```python
from build123d import *

# Parameters (mm, degrees)
BASPROSKE_W        = 10
BASPROSKE_H        = 22.5
TOOTHCUT_DEPTH     = 34.35416016
TEETHCUTS_COUNT    = 28
TEETHCUTS_ANGLE    = 347.142857143
BORSKE_R           = 7.5
BORE_DEPTH         = 50.0000508
CROQUIS1_OUTSIDE_W = 59.636
CROQUIS1_OUTSIDE_H = 59.636
EXTRUIR1_DEPTH     = 10
CROQUIS2_R         = 7.5
CROQUIS2_R_2       = 3.1
EXTRUIR2_DEPTH     = 10
REDONDEO1_R        = 3


with BuildPart() as part:
    # BasProSke → Base-Revolve (revolve)
    with BuildSketch(Plane(origin=(0, 0, 0), x_dir=(1, 0, 0), z_dir=(0, 1, 0)), mode=Mode.PRIVATE) as base_revolve_sk:
        with Locations((5, 11.25)):
            Rectangle(BASPROSKE_W, BASPROSKE_H)
    revolve(base_revolve_sk.sketch.rotate(Axis((-10, 0, 0), (1, 0, 0)), 180), axis=Axis((-10, 0, 0), (1, 0, 0)))

    # TooCutSke → ToothCut (cut, through all)
    with BuildSketch(Plane(origin=(0, 0, 0), x_dir=(0, 0, -1), z_dir=(1, 0, 0))):
        with BuildLine():
            ThreePointArc((0.70071741, 19.111158288), (0, 19.124), (-0.70071741, 19.111158288))
            ThreePointArc((-0.70071741, 19.111158288), (-1.220048441, 20.845037035), (-2.098754998, 22.427413418))
            ThreePointArc((-2.098754998, 22.427413418), (0, 22.5254), (2.098754998, 22.427413418))
            ThreePointArc((2.098754998, 22.427413418), (1.220048441, 20.845037035), (0.70071741, 19.111158288))
        make_face()
    toothcut = extrude(amount=TOOTHCUT_DEPTH, mode=Mode.SUBTRACT)

    # TeethCuts: ToothCut ×28 about axis
    teethcuts_axis = Axis((-10, 0, 0), (1, 0, 0))
    for i in range(1, TEETHCUTS_COUNT):
        add(toothcut.rotate(teethcuts_axis, i * TEETHCUTS_ANGLE / (TEETHCUTS_COUNT - 1)), mode=Mode.SUBTRACT)

    # BorSke → Bore (cut, symmetric)
    with BuildSketch(Plane(origin=(0, 0, 0), x_dir=(0, 0, -1), z_dir=(1, 0, 0))):
        with Locations(Location((0, 0, 0), (0, 0, 180))):
            Circle(BORSKE_R)
    extrude(amount=BORE_DEPTH, both=True, mode=Mode.SUBTRACT)

    # Croquis1 outside → Extruir1 (cut)
    with BuildSketch(Plane(origin=(10, 0, 0), x_dir=(0, 0, -1), z_dir=(1, 0, 0))):
        Rectangle(CROQUIS1_OUTSIDE_W, CROQUIS1_OUTSIDE_H)
        with BuildLine():
            Line((0, 19.124), (0, 0))
            Line((0, 0), (19.124, 0))
            ThreePointArc((19.124, 0), (29.041866068, 29.041866068), (0, 19.124))
        make_face(mode=Mode.SUBTRACT)
    extrude(amount=-EXTRUIR1_DEPTH, mode=Mode.SUBTRACT)

    # Croquis2 → Extruir2 (add, through all)
    with BuildSketch(Plane(origin=(10, 0, 0), x_dir=(0, 0, -1), z_dir=(1, 0, 0))):
        Circle(CROQUIS2_R)
        Circle(CROQUIS2_R_2, mode=Mode.SUBTRACT)
    extrude(amount=-EXTRUIR2_DEPTH)

    # Redondeo1
    redondeo1_edges = [part.edges().sort_by_distance(p)[0] for p in [
        (5, 7.5, 0),
        (5, 0, -7.5),
    ]]
    fillet(redondeo1_edges, radius=REDONDEO1_R)


solid = part.part
```
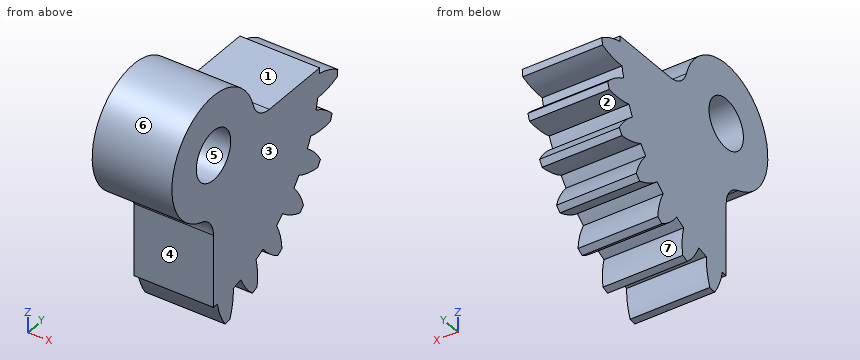
Part model, mm, in its own coordinate system. Face numbers are marked on the shaded views. A direction names the side the tool comes from. Round coordinates to 2 decimals unless told otherwise and drop trailing zeros. Order: outer loops, then holes, each group sorted by start corner. A loop starts at its lowest first (then second) coordinate and runs counter-clockwise, first axis right, second up. Notation, with made-up numbers: M 31,39 L 78,39 A15 ccw 78,63 Z; hole C 1.25,-2.5 d6. An arc over 180 degrees is marked long. Put each result on its own line as item: value. Start each with the question number.
1. Drop flat-ended pins along their axis: pin 1 (4.5 mm diameter, centred on x = 4, y = 14, fed in from +Z); pin 2 (6 mm diameter, centred on x = 3, y = 6.5, fed in from +Z); pin 3 (2 mm diameter, centred on x = 8, y = 9, fed in from +Z); pin 4 (2 mm diameter, centred on x = 9, y = 3, fed in from -Z). Give the stop position or say it passes through.
2. Slice it at B-B on y = 15. List the corners of the cut face in (x, z), then the cut area to 3 significant figures.
3. Tool access for the marked faces 1, 2 and 3: list every direction of +Z, -Z, +X, -X, +Y, -Y with a clear straight run to the whole face (end or side of a thin tool).
4. Drill centre lines: probe 1 along Y at (x, z) = (5.5, -2); probe 2 along Z at (x, y) = (9.75, 2.5); probe 3 along Y at (x, z) = (0.75, -15.5). Where is each one in solid material? Low to high. Write a range as [from, to].
5. Slice it at C-C on y = 6.25. List the corners of the cut face in (x, z).
6. Slice it at D-D on z = -13.5. List the corners of the cut face in (x, y).
7. Slice it at A-A on z = 0.75. List the corners of the cut face in (x, y), then the cut area to 3 significant figures.
8. Two-plate mould, pull along Z, no slides. Class the marked faces 4, 5, 6 and 7: +Z half, -Z half, draft (parallel to the pull), parting line (faces both ways), or undercut.
Findings:
1. pin 1: z = 0
1. pin 2: z = 6.63
1. pin 3: z = 0.82
1. pin 4: z = -22.4
2. outline: M 0,-16.02 L 10,-16.02 L 10,-13.09 L 0,-13.09 Z; M 0,-11.86 L 10,-11.86 L 10,0 L 0,0 Z
2. area: 148 mm2
3. face 1: +Z, +X, -X, +Y
3. face 2: +X, -X
3. face 3: +Z, -Z, +X, +Y, -Y
4. probe 1: [-7.23, -2.37], [2.37, 22.28]
4. probe 2: [-22.36, -1.83], [1.83, 7.07]
4. probe 3: [0, 11.43], [13.88, 16.19]
5. outline: M 0,-20.59 L 10,-20.59 L 10,4.15 L 0,4.15 Z
6. outline: M 0,0 L 10,0 L 10,15.27 L 0,15.27 Z
7. outline: M 0,-7.46 L 10,-7.46 L 10,-3.01 L 0,-3.01 Z; M 0,3.01 L 10,3.01 L 10,8.08 L 0,8.08 Z
7. area: 95.2 mm2
8. face 4: draft
8. face 5: undercut
8. face 6: parting line
8. face 7: undercut
